Read the model definition and answer for the solid it produces. Units are mm, in the model's axes. Face numbers are marked on the shaded views. A direction names the side the tool comes from. Round coordinates to 2 decimals unless told otherwise and drop trailing zeros. Write each loop counter-clockwise with the first axis right and the second up, starting at its lowest first coordinate (ties: lowest second). Pieces come first, ordered by that corner, then holes.
from build123d import *

# Parameters (mm, degrees)
M8X1_0_TAPPED_HOLE1_D = 7
SKETCH6_R             = 1.25
SKETCH6_W             = 17.472275608
SKETCH6_H             = 29.884909838
SKETCH6_W_2           = 8.845933312
CUT_EXTRUDE1_DEPTH    = 3.5


with BuildPart() as part:
    # Sketch1 → Revolve1 (revolve)
    with BuildSketch(Plane.XY):
        Polygon((0, 0), (0, 5), (4.5, 5), (4.5, 12), (8, 12), (8, 5), (10, 5), (10, 0), align=None)
    revolve(axis=Axis((-27.226239534, 0, 0), (1, 0, 0)))

    # M8x1.0 Tapped Hole1 (through all)
    with Locations(Plane(origin=(10, 0, 0), x_dir=(0, 0, -1), z_dir=(1, 0, 0))):
        with Locations((0, 0)):
            Hole(M8X1_0_TAPPED_HOLE1_D / 2)

    # Sketch6 → Cut-Extrude1 (cut)
    with BuildSketch(Plane(origin=(8, 0, 0), x_dir=(0, 0, -1), z_dir=(1, 0, 0))):
        with Locations((0, 8.75)):
            Circle(SKETCH6_R)
        with Locations((0, -8.75)):
            Circle(SKETCH6_R)
        with Locations((13.986137804, 0)):
            Rectangle(SKETCH6_W, SKETCH6_H)
        with Locations((-9.672966656, 0)):
            Rectangle(SKETCH6_W_2, SKETCH6_H)
    extrude(amount=-CUT_EXTRUDE1_DEPTH, mode=Mode.SUBTRACT)


solid = part.part
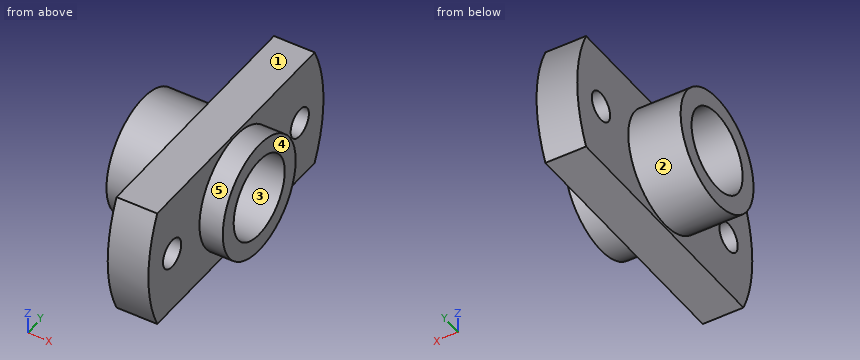
Q1. Which of the six approach directions +Z, -Z, +X, -X, +Y, -Y give full straight-line access (tool end or side, diameter ignored) to the marked faces 1 and 2?
Verdict:
face 1: +Z, +X, -X, +Y, -Y
face 2: -X
Q2. Flat-ended cylindrical pins translate along their axes: pin 1 Ø1.5 at (y, z) = (-9, -1.5) entering from +X; pin 2 Ø3 at (y, z) = (-8.75, 0) entering from -X. Find the tip coordinate at first contact, or state that the pin passes through.
Verdict:
pin 1: stops at x = 8
pin 2: stops at x = 4.5
Q3. Section D-D (x = 2.75) is taken. Determine the outline of the cut face in (y, z), then the cut area to 3 significant figures.
Verdict:
outline: circle Ø10 at (0, 0); hole circle Ø7 at (0, 0)
area: 40.1 mm2
Q4. Determine the mould class of the marked faces 3, 4 and 5 for opening direction Y: pulls with the +Y half, pulls with the -Y half, needs draft (parallel to the pull), parting line crosses it, or undercut.
Verdict:
face 3: undercut
face 4: needs draft
face 5: parting line crosses it
Q5. Straight lines are drawn through the part: probe 1 along Y at (x, z) = (6, 0); probe 2 along X at (y, z) = (-10, 4); probe 3 along Y at (x, z) = (6.75, 2.25). For each, find the intervals that lie inside material, in ascending order.
Verdict:
probe 1: y = -12 to -10, -7.5 to -3.5, 3.5 to 7.5, 10 to 12
probe 2: x = 4.5 to 8
probe 3: y = -11.79 to -2.68, 2.68 to 11.79
Q6. Section A-A (y = 0) is taken. Determine the outline of the cut face in (x, z).
Verdict:
outline: (0, -5) - (4.5, -5) - (4.5, -5.25) - (8, -5.25) - (8, -5) - (10, -5) - (10, -3.5) - (0, -3.5) - close; (0, 3.5) - (10, 3.5) - (10, 5) - (8, 5) - (8, 5.25) - (4.5, 5.25) - (4.5, 5) - (0, 5) - close
Q7. Section B-B (z = 0) is taken. Determine the outline of the cut face in (x, y), then the cut area to 3 significant figures.
Verdict:
outline: (0, -5) - (4.5, -5) - (4.5, -7.5) - (8, -7.5) - (8, -5) - (10, -5) - (10, -3.5) - (0, -3.5) - close; (0, 3.5) - (10, 3.5) - (10, 5) - (8, 5) - (8, 7.5) - (4.5, 7.5) - (4.5, 5) - (0, 5) - close; (4.5, -12) - (8, -12) - (8, -10) - (4.5, -10) - close; (4.5, 10) - (8, 10) - (8, 12) - (4.5, 12) - close
area: 61.5 mm2
Q8. Section C-C (x = 7.5) is taken. Determine the outline of the cut face in (y, z), then the cut area to 3 significant figures.
Verdict:
outline: (-10.79, -5.25) - (10.79, -5.25) arc R12 ccw to (10.79, 5.25) - (-10.79, 5.25) arc R12 ccw to start; hole circle Ø2.5 at (-8.75, 0); hole circle Ø7 at (0, 0); hole circle Ø2.5 at (8.75, 0)
area: 195 mm2
